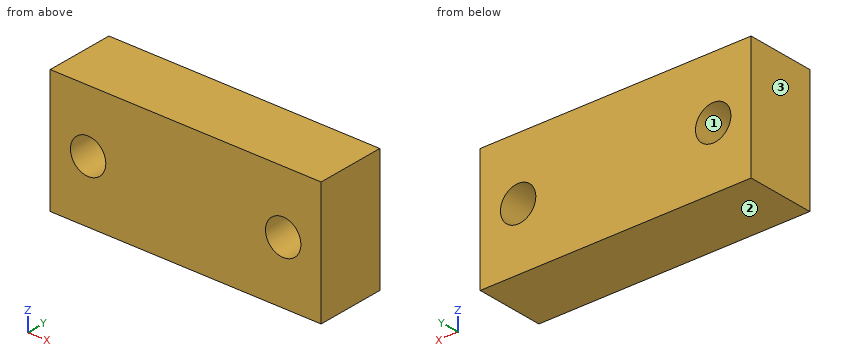
Autodesk Inventor part; units mm, degrees
ref_plane "YZ Plane" through (0, 0, 0) normal (1, 0, 0) x (0, 1, 0)
ref_plane "XZ Plane" through (0, 0, 0) normal (0, 1, 0) x (-1, 0, 0)
ref_plane "XY Plane" through (0, 0, 0) normal (0, 0, 1) x (1, 0, 0)
sketch "Sketch4" plane through (0, 0, 0) normal (0, 1, 0) x (-1, 0, 0)
  line L0 (-12.5, -5.708) -> (12.5, -5.708)
  line L1 (12.5, -5.708) -> (12.5, 5.708)
  line L2 (12.5, 5.708) -> (-12.5, 5.708)
  line L3 (-12.5, 5.708) -> (-12.5, -5.708)
  line L4 (-12.5, -5.708) -> (12.5, 5.708) construction
  line L5 (12.5, -5.708) -> (-12.5, 5.708) construction
  point P0 (0, 0)
  dimension "d22" = 11.416
  dimension "d23" = 25
extrude "Extrusion3" add sketch "Sketch4" along normal mid plane 6.35
sketch "Sketch5" plane through (0, 3.175, 0) normal (0, 1, 0) x (1, 0, 0)
  line L0 (12.5, 5.708) -> (-12.5, 5.708)
  line L1 (-12.5, 5.708) -> (-12.5, -5.708)
  line L2 (-12.5, -5.708) -> (12.5, -5.708)
  line L3 (12.5, -5.708) -> (12.5, 5.708)
  line L4 (9, 0) -> (0, 0)
  dimension "d26" = 9
hole "Hole2" at (9, 3.175, 0) direction (0, -1, 0) diameter 3.264 end through all
mirror "Mirror2" about plane through (0, 0, 0) normal (1, 0, 0) of "Hole2"
equation "\"d22\" = 2 * silveringThickness + ScintillatorThickness + 2 * rubberizedCoating"
equation "\"d26\" = MountingScrewOffsett"
equation "\"OpticalFiberClearence\" = 0.071"
equation "\"ScintillatorEdgeClearence\" = 3"
equation "\"ShallowTrackDepth\" = 1.142"
equation "\"DeepTrackDepth\" = 5.571"
equation "\"FiberEdgeOffsett\" = 5"
equation "\"LoopLargeTrackRatio\" = 1.1"
equation "\"FiberSensorClerence\" = 0.5"
equation "\"MountingScrewOffsett\" = 9"
equation "\"silveringThickness\" = 0.2"
equation "\"mppcMountDepth\" = 6.35"
properties part number "suppourtBlock" material "Aluminum 6061"
Part model, mm, in its own coordinate system. Face numbers are marked on the shaded views. Round coordinates to 2 decimals unless told otherwise and drop trailing zeros. Write each loop counter-clockwise with the first axis right and the second up, starting at its lowest first coordinate (ties: lowest second). Pieces come first, ordered by that corner, then holes. Notation, with made-up numbers: (55.5, -32.75) - (102.5, -32.75) arc R22 cw to (102.5, -20.75) - close; hole circle Ø2 at (-15.75, -13.5). An arc over 180 degrees is marked (long way). Use CSV: the item, a comma, the result in double quotes.
Item 1: Pull direction Z, two halves, no side cores. Call the marked faces 1, 2 and 3: pulls with the +Z half, pulls with the -Z half, needs draft (parallel to the pull), parting line crosses it, or undercut.
Results list:
face 1,"undercut"
face 2,"pulls with the -Z half"
face 3,"needs draft"
Item 2: Slice it at C-C, the plane y = 0.5. Write the cut outline in (x, z), then the cut area to 3 significant figures.
Results list:
outline,"(-12.5, -5.71) - (12.5, -5.71) - (12.5, 5.71) - (-12.5, 5.71) - close; hole circle Ø3.26 at (-9, 0); hole circle Ø3.26 at (9, 0)"
area,"269 mm²"
Item 3: Flat gauge pin, fed straight in: P1, Ø3, axis at x = -9, z = 0, coming from the +Y side. Where does the tip first touch, or does it go through?
Results list:
P1,"passes through"
Item 4: Wall check: L1, parallel to X at y = -1.25, z = 0; L2, parallel to Z at x = -9, y = 0.5. Give the ranges that are in metal, low to high.
Results list:
L1,"x = -12.5 to -10.63, -7.37 to 7.37, 10.63 to 12.5"
L2,"z = -5.71 to -1.63, 1.63 to 5.71"
Item 5: Slice it at B-B, the plane x = -9. Write the cut outline in (y, z) (3 decimals).
Results list:
outline,"(-3.175, -5.708) - (3.175, -5.708) - (3.175, -1.632) - (-3.175, -1.632) - close; (-3.175, 1.632) - (3.175, 1.632) - (3.175, 5.708) - (-3.175, 5.708) - close"
Item 6: Slice it at A-A, the plane z = 0. Write the cut outline in (x, y) (3 decimals), then the cut area to 3 significant figures.
Results list:
outline,"(-12.5, -3.175) - (-10.632, -3.175) - (-10.632, 3.175) - (-12.5, 3.175) - close; (-7.368, -3.175) - (7.368, -3.175) - (7.368, 3.175) - (-7.368, 3.175) - close; (10.632, -3.175) - (12.5, -3.175) - (12.5, 3.175) - (10.632, 3.175) - close"
area,"117 mm²"
